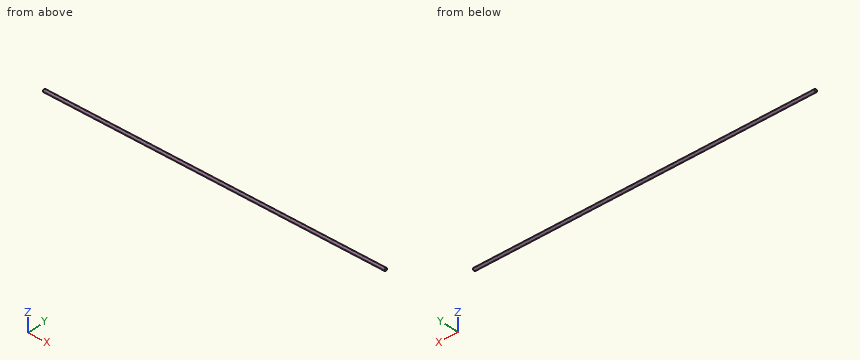
Autodesk Inventor part; units mm, degrees
ref_plane "YZ Plane" through (0, 0, 0) normal (1, 0, 0) x (0, 1, 0)
ref_plane "XZ Plane" through (0, 0, 0) normal (0, 1, 0) x (-1, 0, 0)
ref_plane "XY Plane" through (0, 0, 0) normal (0, 0, 1) x (1, 0, 0)
sketch "Sketch1" plane through (0, 0, 0) normal (0, 1, 0) x (-1, 0, 0)
  arc A0 (-4, 0) -> (0, 0) centre (-2, 0.1626) ccw
  line L0 (0, 0) -> (-4, 0)
sketch "Sketch2" plane through (0, 0, 0) normal (1, 0, 0) x (0, 1, 0)
  line L0 (0, 0) -> (-2.0066, 0)
  line L1 (-2.0066, 0) -> (-2.0066, -2.0066)
  line L2 (-2.0066, -2.0066) -> (0, -2.0066)
  line L3 (0, -2.0066) -> (0, 0)
  dimension "d0" = 2.0066
  dimension "d1" = 2.0066
extrude "Extrusion1" add sketch "Sketch2" against normal blind 250
fillet "Fillet1" radius 0.9906 4 edges at (-125, 0, 0) (-125, -2.0066, 0) (-125, 0, -2.0066) (-125, -2.0066, -2.0066)
properties part number "LeverArm" material "Stainless Steel"
Can you work these out from the model? Positions are in its coordinate system, mm. Round coordinates to 2 decimals unless told otherwise and drop trailing zeros. Write each loop counter-clockwise with the first axis right and the second up, starting at its lowest first coordinate (ties: lowest second). Pieces come first, ordered by that corner, then holes. Notation, with made-up numbers: (81.5, -22) -> (126.5, -22) arc R12 ccw to (126.5, -7) -> close; hole circle Ø8 at (81.25, 14). An arc over 180 degrees is marked (long way). One line per question, with ' | ' between items. Start each with the question number.
1) Suppose I cut it at B-B on z = -1.4. Write out the boundary of the cut face in (x, y).
2) Suppose I cut it at C-C on y = -1.6. Write out the boundary of the cut face in (x, z), then the cut area to 3 significant figures.
3) I need wall thicknesses on line 1 (Y direction, x = -72.5, z = -0.9); line 2 (Z direction, x = -214, y = -0.75); line 3 (Z direction, x = -198, y = -0.1). Which ranges of each line are inside material? Lowest first, please. Write a range as [from, to].
Return value:
1) outline: (-250, -1.93) -> (0, -1.93) -> (0, -0.08) -> (-250, -0.08) -> close
2) outline: (-250, -1.82) -> (0, -1.82) -> (0, -0.19) -> (-250, -0.19) -> close | area: 406 mm2
3) line 1: y = [-2, 0] | line 2: z = [-1.98, -0.03] | line 3: z = [-1.45, -0.56]
